from build123d import *

# Parameters (mm, degrees)
SKETCH1_R            = 42.5
SKETCH1_R_2          = 27.5
BOSS_EXTRUDE1_DEPTH  = 1
M6_CLEARANCE_HOLE1_D = 7


with BuildPart() as part:
    # Sketch1 → Boss-Extrude1 (new body)
    with BuildSketch(Plane.XY):
        Circle(SKETCH1_R)
        Circle(SKETCH1_R_2, mode=Mode.SUBTRACT)
    extrude(amount=BOSS_EXTRUDE1_DEPTH)

    # M6 Clearance Hole1 (through all)
    with Locations(Plane.XY.offset(1)):
        with Locations((-33.875, 0), (-16.9375, -29.336610553), (16.9375, -29.336610553), (33.875, 0), (16.9375, 29.336610553), (-16.9375, 29.336610553)):
            Hole(M6_CLEARANCE_HOLE1_D / 2)


solid = part.part
Verification items for the finished model (mm, model axes). Give positions to 0.01 mm unless a question says otherwise; leave off trailing zeros. Write each loop counter-clockwise with the first axis right and the second up, starting at its lowest first coordinate (ties: lowest second). Pieces come first, ordered by that corner, then holes. Notation, with made-up numbers: (81, 52) - (117, 52) arc R26 cw to (117, 89) - close; hole circle Ø5 at (60, 75). An arc over 180 degrees is marked (long way). Answer as CSV lines item,"result". Start each with the question number.
1. Thickness scan on line 1 (X direction, y = 2.5, z = 0.65); line 2 (X direction, y = 32.5, z = 0.75); line 3 (Y direction, x = 19.5, z = 0.4). Record the ranges inside material, lowest first.
2. Sectioned sample at C-C (z = 0.5). Record the boundary of the cut face in (x, y) (1 decimal), then the cut area to 3 significant figures.
3. Draft check along X on faces 1 (the face through (-1, -28, 1)), 2 (the face through (36.65, -2.13, 0.49)), 3 (the face through (-33.727, -25.861, 0.493)). Enter one of: pulls with the +X half, pulls with the -X half, needs draft (parallel to the pull), parting line crosses it, or undercut.
4. Depth check by flat-ended pin: pin 1 (5.5 mm diameter, centred on x = -16.94, y = 29.34, fed in from -Z). Enter the tip coordinate at first touch or a pass-through.
5. Sectioned sample at A-A (x = 0). Record the boundary of the cut face in (y, z), then the cut area to 3 significant figures.
6. Sectioned sample at B-B (y = 0). Record the boundary of the cut face in (x, z) (3 decimals), then the cut area to 3 significant figures.
7. Sectioned sample at D-D (y = 18.5). Record the boundary of the cut face in (x, z).
Derived:
1,line 1,"-42.43 to -36.32, -31.43 to -27.39, 27.39 to 31.43, 36.32 to 42.43"
1,line 2,"-27.39 to -18.44, -15.44 to 15.44, 18.44 to 27.39"
1,line 3,"-37.76 to -31.72, -26.95 to -19.39, 19.39 to 26.95, 31.72 to 37.76"
2,outline,"circle Ø85 at (0, 0); hole circle Ø7 at (-33.9, 0); hole circle Ø55 at (0, 0); hole circle Ø7 at (-16.9, -29.3); hole circle Ø7 at (-16.9, 29.3); hole circle Ø7 at (16.9, -29.3); hole circle Ø7 at (16.9, 29.3); hole circle Ø7 at (33.9, 0)"
2,area,"3,070 mm²"
3,face 1,"needs draft"
3,face 2,"undercut"
3,face 3,"parting line crosses it"
4,pin 1,"through"
5,outline,"(-42.5, 0) - (-27.5, 0) - (-27.5, 1) - (-42.5, 1) - close; (27.5, 0) - (42.5, 0) - (42.5, 1) - (27.5, 1) - close"
5,area,"30.0 mm²"
6,outline,"(-42.5, 0) - (-37.375, 0) - (-37.375, 1) - (-42.5, 1) - close; (-30.375, 0) - (-27.5, 0) - (-27.5, 1) - (-30.375, 1) - close; (27.5, 0) - (30.375, 0) - (30.375, 1) - (27.5, 1) - close; (37.375, 0) - (42.5, 0) - (42.5, 1) - (37.375, 1) - close"
6,area,"16.0 mm²"
7,outline,"(-38.26, 0) - (-20.35, 0) - (-20.35, 1) - (-38.26, 1) - close; (20.35, 0) - (38.26, 0) - (38.26, 1) - (20.35, 1) - close"
